For this review, take the finished solid that the model builds, in its own axes (mm). A direction names the side the tool comes from. Coordinates: 2 decimals unless noted, no trailing zeros. Order: outer loops, then holes, each group sorted by start corner. A loop starts at its lowest first (then second) coordinate and runs counter-clockwise, first axis right, second up. Notation, with made-up numbers: M -15.5,-25.75 L -7.5,-25.75 A18 ccw -7.5,-7.75 Z; hole C 75,39 d7. An arc over 180 degrees is marked long. Use CSV: the item, a comma, the result in double quotes.
Autodesk Inventor part; units mm, degrees
ref_plane "YZ Plane" through (0, 0, 0) normal (1, 0, 0) x (0, 1, 0)
ref_plane "XZ Plane" through (0, 0, 0) normal (0, 1, 0) x (-1, 0, 0)
ref_plane "XY Plane" through (0, 0, 0) normal (0, 0, 1) x (1, 0, 0)
sketch "スケッチ1" plane through (0, 0, 0) normal (0, 0, 1) x (1, 0, 0)
  line L0 (0, 0) -> (18, 0)
  line L1 (18, 0) -> (18, 18)
  line L2 (18, 18) -> (0, 18)
  line L3 (0, 18) -> (0, 0)
  line L4 (0, 13.7574) -> (4.2426, 18)
  line L5 (0, 13.7574) -> (6, 13.7574) construction
  line L6 (4.2426, 0) -> (0, 4.2426)
  line L7 (18, 4.2426) -> (13.7574, 0)
  line L8 (13.7574, 18) -> (18, 13.7574)
  point P0 (0, 9)
  point P1 (9, 18)
  point P2 (9, 9)
  dimension "d0" = 18
  dimension "d1" = 18
  dimension "d2" = 45
  dimension "d3" = 3
  dimension "d13" = 9
  dimension "d14" = 9
  dimension "d17" = 360
extrude "押し出し1" add sketch "スケッチ1" along normal blind 9.5 contours L6 L3 L4 L2 L8 L1 L7 L0
sketch "スケッチ2" plane through (0, 0, 9.5) normal (0, 0, 1) x (1, 0, 0)
  line L0 (0, 0) -> (13.7574, 0)
  line L1 (0, 13.7574) -> (0, 0)
  circle A0 centre (9, 9) radius 8.7
  point P0 (9, 0)
  point P1 (5.6569, 0)
  point P2 (12.3431, 0)
  point P3 (0, 9.7071)
  point P4 (0, 5.6569)
  point P5 (18, 0)
  point P6 (0, 18)
  dimension "d10" = 17.4
extrude "押し出し2" add sketch "スケッチ2" along normal blind 85
sketch "スケッチ3" plane through (9, 9, 94.5) normal (0, 0, 1) x (1, 0, 0)
  circle A0 centre (0, 0) radius 8.7
  line L0 (4.7574, 9) -> (-4.7574, 9)
  line L1 (-4.7574, 9) -> (-9, 4.7574)
  line L2 (-9, 4.7574) -> (-9, -4.7574)
  line L3 (-9, -4.7574) -> (-4.7574, -9)
  line L4 (-4.7574, -9) -> (4.7574, -9)
  line L5 (4.7574, -9) -> (9, -4.7574)
  line L6 (9, -4.7574) -> (9, 4.7574)
  line L7 (9, 4.7574) -> (4.7574, 9)
  point P0 (-9, -9)
extrude "押し出し3" add sketch "スケッチ3" along normal blind 12.5 contours A0 | L7 L6 L5 L4 L3 L2 L1 L0
sketch "スケッチ4" plane through (9, 9, 107) normal (0, 0, 1) x (1, 0, 0)
  circle A0 centre (0, 0) radius 8.7
  circle A1 centre (0, 0) radius 6
  point P0 (-9, -9)
  dimension "d21" = 12
extrude "押し出し4" add sketch "スケッチ4" along normal blind 8 contours A1
sketch "スケッチ5" plane through (9, 9, 115) normal (0, 0, 1) x (1, 0, 0)
  circle A0 centre (0, 0) radius 6
  circle A1 centre (0, 0) radius 3
  point P0 (-9, -9)
  dimension "d24" = 6
extrude "押し出し5" cut sketch "スケッチ5" against normal blind 70 contours A1
properties part number "airclinder_60" material "アルミニウム 6061-AHC"
Item 1: To check wall thickness, follow line 1 along Y through (x, z) = (9, 70.5); line 2 along Z through (x, y) = (17, 14); line 3 along Z through (x, y) = (3.25, 6.75). State the ranges of each line that lie inside material, in increasing order. Write a range as [from, to].
Solutions:
line 1,"[0.3, 6], [12, 17.7]"
line 2,"[0, 9.5], [94.5, 107]"
line 3,"[0, 107]"
Item 2: Clearance check with flat-ended pins moving along their axes: pin 1 Ø6 at (y, z) = (5.5, 19.5) entering from +X; pin 2 Ø5 at (y, z) = (9, 56) entering from -X; pin 3 Ø10 at (x, z) = (10, 77) entering from -Y. State where each tip first meets the part, or that it passes through.
Solutions:
pin 1,"x = 17.69"
pin 2,"x = 0.3"
pin 3,"y = 0.3"
Item 3: Add section A-A on y = 9. State the section outline as (x, z) points, and give its area (3 significant figures).
Solutions:
outline,"M 0,0 L 18,0 L 18,9.5 L 17.7,9.5 L 17.7,94.5 L 18,94.5 L 18,107 L 15,107 L 15,115 L 12,115 L 12,45 L 6,45 L 6,115 L 3,115 L 3,107 L 0,107 L 0,94.5 L 0.3,94.5 L 0.3,9.5 L 0,9.5 Z"
area,"1,550 mm^2"
Item 4: Add section B-B on z = 85. State the section outline as (x, y) points.
Solutions:
outline,"C 9,9 d17.4; hole C 9,9 d6"
Item 5: Add section C-C on x = 16. State the section outline as (y, z) points, and give its area (3 significant figures).
Solutions:
outline,"M 2.24,0 L 15.76,0 L 15.76,9.5 L 14.17,9.5 L 14.17,94.5 L 15.76,94.5 L 15.76,107 L 2.24,107 L 2.24,94.5 L 3.83,94.5 L 3.83,9.5 L 2.24,9.5 Z"
area,"1,180 mm^2"
Item 6: Add section D-D on z = 27.5. State the section outline as (x, y) points, and give its area (3 significant figures).
Solutions:
outline,"C 9,9 d17.4"
area,"238 mm^2"
Item 7: For faces 1 (the face through (11, 3, 107)), 2 (the face through (2.59, 3.12, 51.4)), 3 (the face through (18, 9, 101)), list the 3-axis set-ups (+Z, -Z, +X, -X, +Y, -Y) from which the entire face can be reached by the end or side of a thin tool; tool diameter is ignored.
Solutions:
face 1,"+Z"
face 2,"none"
face 3,"+Z, -Z, +X, +Y, -Y"
